Verification items for the finished model (mm, model axes). Face numbers are marked on the shaded views. A direction names the side the tool comes from. Round coordinates to 2 decimals unless told otherwise and drop trailing zeros. Write each loop counter-clockwise with the first axis right and the second up, starting at its lowest first coordinate (ties: lowest second). Pieces come first, ordered by that corner, then holes. Notation, with made-up numbers: (85, 69.25) -> (134, 69.25) arc R22 cw to (134, 92.25) -> close; hole circle Ø7 at (-36.75, 6.5). An arc over 180 degrees is marked (long way). Use CSV: the item, a comma, the result in double quotes.
```python
from build123d import *

# Parameters (mm, degrees)
SKETCH1_R           = 2
SKETCH1_R_2         = 13.5
BOSS_EXTRUDE1_DEPTH = 7.5
SKETCH2_R           = 2.6
CUT_EXTRUDE1_DEPTH  = 20
SKETCH4_R           = 2.5
CUT_EXTRUDE2_DEPTH  = 10
SKETCH2_3_R         = 2.6
CUT_EXTRUDE3_DEPTH  = 54.677276398


with BuildPart() as part:
    # Sketch1 → Boss-Extrude1 (new, symmetric)
    with BuildSketch(Plane(origin=(0, 0, 0), x_dir=(0, 0, -1), z_dir=(1, 0, 0))):
        with BuildLine():
            Line((24.999999999, 35), (9.721359549, 35))
            ThreePointArc((9.721359549, 35), (5.126301138, 34.464979789), (0.777087639, 32.88854382))
            Line((0.777087639, 32.88854382), (-3.944271911, 30.527864045))
            ThreePointArc((-3.944271911, 30.527864045), (-12.013016168, 23.153942467), (-15.000000001, 12.639320225))
            Line((-15.000000001, 12.639320225), (-15.000000001, -12.639320225))
            ThreePointArc((-15.000000001, -12.639320225), (-12.013016168, -23.153942467), (-3.944271911, -30.527864045))
            Line((-3.944271911, -30.527864045), (0.777087639, -32.88854382))
            ThreePointArc((0.777087639, -32.88854382), (5.126301138, -34.464979789), (9.721359549, -35))
            Line((9.721359549, -35), (24.999999999, -35))
            Line((24.999999999, -35), (24.999999999, 35))
        make_face()
        with Locations((0, 18.25)):
            Circle(SKETCH1_R, mode=Mode.SUBTRACT)
        Circle(SKETCH1_R_2, mode=Mode.SUBTRACT)
        with Locations(Location((0, -18.25, 0), (0, 0, 180))):
            Circle(SKETCH1_R, mode=Mode.SUBTRACT)
    extrude(amount=BOSS_EXTRUDE1_DEPTH, both=True)

    # Sketch2 → Cut-Extrude1 (cut)
    # profile 1 of 2: a face of its own
    with BuildSketch(Plane.XY.offset(15.000000001)):
        Polygon((0, -22.765727793), (-4.1, -25.132863896), (-4.1, -29.867136104), (0, -32.234272207), (4.1, -29.867136104), (4.1, -25.132863896), align=None)
        with Locations((0, -27.5)):
            Circle(SKETCH2_R, mode=Mode.SUBTRACT)
    # profile 2 of 2: a face of its own
    with BuildSketch(Plane.XY.offset(15.000000001)):
        Polygon((0, 32.234272207), (-4.1, 29.867136104), (-4.1, 25.132863896), (0, 22.765727793), (4.1, 25.132863896), (4.1, 29.867136104), align=None)
        with Locations((0, 27.5)):
            Circle(SKETCH2_R, mode=Mode.SUBTRACT)
    extrude(amount=-CUT_EXTRUDE1_DEPTH, mode=Mode.SUBTRACT)

    # Sketch4 → Cut-Extrude2 (cut)
    with BuildSketch(Plane.XY.offset(15.000000001)):
        Circle(SKETCH4_R)
    extrude(amount=-CUT_EXTRUDE2_DEPTH, mode=Mode.SUBTRACT)

    # Sketch2_3 → Cut-Extrude3 (cut, through all)
    with BuildSketch(Plane.XY.offset(15.000000001)):
        with Locations((0, 27.5)):
            Circle(SKETCH2_3_R)
        with Locations((0, -27.5)):
            Circle(SKETCH2_3_R)
    extrude(amount=-CUT_EXTRUDE3_DEPTH, mode=Mode.SUBTRACT)


solid = part.part
```
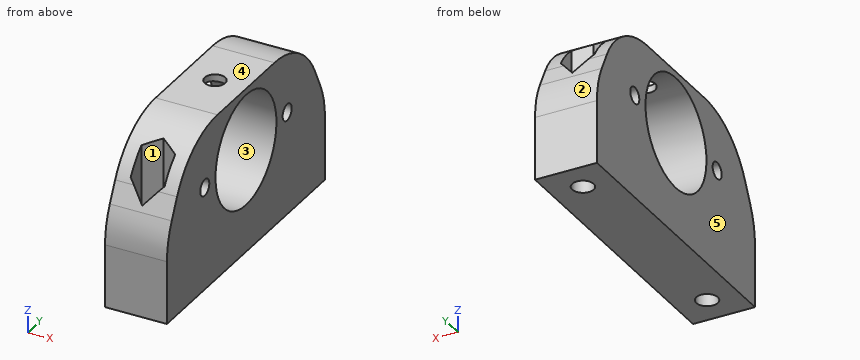
Q1. Material ranges on L1, parallel to Y at x = 0, z = -20; L2, parallel to Y at x = -2, z = -22; L3, parallel to Y at x = -4, z = 3, recorded low to high.
Filled in:
L1,"-35 to -30.1, -24.9 to 24.9, 30.1 to 35"
L2,"-35 to -29.16, -25.84 to 25.84, 29.16 to 35"
L3,"-31 to -29.92, -25.08 to -13.16, 13.16 to 25.08, 29.92 to 31"
Q2. Section check A-A (y = 0). Record the cut outline in (x, z), plus the area to 4 significant figures.
Filled in:
outline,"(-7.5, -25) -> (7.5, -25) -> (7.5, -13.5) -> (-7.5, -13.5) -> close; (-7.5, 13.5) -> (-2.5, 13.5) -> (-2.5, 15) -> (-7.5, 15) -> close; (2.5, 13.5) -> (7.5, 13.5) -> (7.5, 15) -> (2.5, 15) -> close"
area,"187.5 mm²"
Q3. Mould release check, pull along Z, two halves, no side actions. Record for the marked faces 3, 4 and 5: released by +Z, released by -Z, zero draft, split by the parting line, or undercut.
Filled in:
face 3,"undercut"
face 4,"released by +Z"
face 5,"zero draft"
Q4. Section check C-C (y = -18.25). Record the cut outline in (x, z), plus the area to 3 significant figures.
Filled in:
outline,"(-7.5, -25) -> (7.5, -25) -> (7.5, -2) -> (-7.5, -2) -> close; (-7.5, 2) -> (7.5, 2) -> (7.5, 14.2) -> (-7.5, 14.2) -> close"
area,"528 mm²"
Q5. Section check D-D (x = 5.75). Record the cut outline in (y, z).
Filled in:
outline,"(-35, -25) -> (35, -25) -> (35, -9.72) arc R20 ccw to (32.89, -0.78) -> (30.53, 3.94) arc R20 ccw to (12.64, 15) -> (-12.64, 15) arc R20 ccw to (-30.53, 3.94) -> (-32.89, -0.78) arc R20 ccw to (-35, -9.72) -> close; hole circle Ø4 at (-18.25, 0); hole circle Ø27 at (0, 0); hole circle Ø4 at (18.25, 0)"
Q6. Access from +Z, -Z, +X, -X, +Y, -Y to the whole of each face (thin tool, end or side, straight path). Record for the marked faces 1 and 2.
Filled in:
face 1,"+Z"
face 2,"+Z, +X, -X, +Y"
Q7. Section check B-B (x = -1). State how many separate pieces and enclosed holes the cut face has, plus the area to 3 significant figures.
Filled in:
separate pieces,"3"
enclosed holes,"2"
area,"1,530 mm²"
Q8. Go/stop test with flat-tipped pins: P1, Ø4, axis at x = -1, z = -5, coming from the +Y side; P2, Ø1, axis at x = 4, y = 22.5, coming from the +Z side; P3, Ø4, axis at x = 0, y = 27.5, coming from the +Z side; P4, Ø2, axis at x = 1.5, z = -4.5, coming from the +Y side. Record where each tip stops, or that it passes through.
Filled in:
P1,"y = 34.81"
P2,"z = 12.67"
P3,"through"
P4,"y = 34.55"
